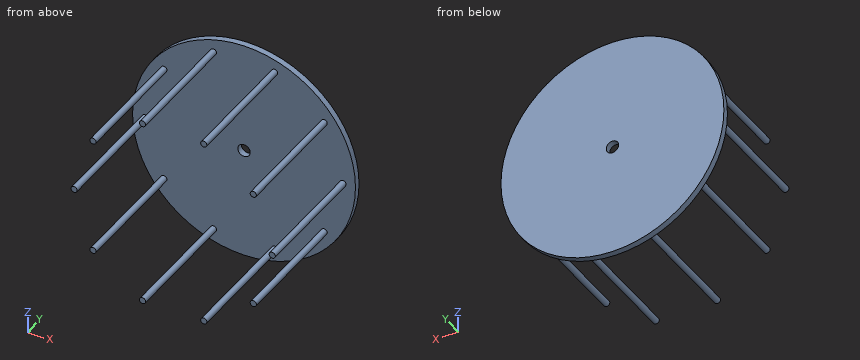
from build123d import *

# Parameters (mm, degrees)
F0_R     = 114.3
F0_R_2   = 6.35
F1_DEPTH = 6.35
F2_R     = 3.175
F3_DEPTH = 127


with BuildPart() as f1:
    # F0 (on Front) → F1 (new body)
    with BuildSketch(Plane.XZ):
        Circle(F0_R)
        Circle(F0_R_2, mode=Mode.SUBTRACT)
    extrude(amount=F1_DEPTH)

    # F2 (on face) → F3 (join)
    with BuildSketch(Plane.XZ.offset(6.35)):
        with Locations((101.6, 0)):
            Circle(F2_R)
        with Locations((82.196127, 59.718982)):
            Circle(F2_R)
        with Locations((31.396127, 96.627342)):
            Circle(F2_R)
        with Locations((-31.396127, 96.627342)):
            Circle(F2_R)
        with Locations((-82.196127, 59.718982)):
            Circle(F2_R)
        with Locations((-101.6, 0)):
            Circle(F2_R)
        with Locations((-82.196127, -59.718982)):
            Circle(F2_R)
        with Locations((-31.396127, -96.627342)):
            Circle(F2_R)
        with Locations((31.396127, -96.627342)):
            Circle(F2_R)
        with Locations((82.196127, -59.718982)):
            Circle(F2_R)
    extrude(amount=F3_DEPTH)


solid = f1.part
Verification items for the finished model (mm, model axes). Give positions to 0.01 mm unless a question says otherwise; leave off trailing zeros. Loops run counter-clockwise (first coordinate to the right, second up) from the corner with the lowest first, then second, coordinate; pieces in that order, holes last.
1) Depth check by flat-ended pin: pin 1 Ø4 at (x, z) = (-78, 17) entering from -Y. Enter the tip coordinate at first touch or a pass-through.
2) Sectioned sample at C-C, the plane y = -22. Count the separate pieces of the cut face and the enclosed holes in it, then the cut area to 3 significant figures.
3) Sectioned sample at B-B, the plane z = 0. Enter the section's corners in (x, y) (3 decimals).
4) Sectioned sample at A-A, the plane x = 0. Enter the section's corners in (y, z), then the cut area to 3 significant figures.
5) Thickness scan on line 1 along Z through (x, y) = (0, -4); line 2 along Y through (x, z) = (100.5, 7); line 3 along Z through (x, y) = (103.5, -14.5). Record the ranges inside material, lowest first.
6) Sectioned sample at D-D, the plane x = -101.6. Enter the section's corners in (y, z) (3 decimals).
Answers:
1. pin 1: stops at y = -6.35
2. separate pieces: 10
2. enclosed holes: 0
2. area: 317 mm2
3. outline: (-114.3, -6.35) - (-104.775, -6.35) - (-104.775, -133.35) - (-98.425, -133.35) - (-98.425, -6.35) - (-6.35, -6.35) - (-6.35, 0) - (-114.3, 0) - close; (6.35, -6.35) - (98.425, -6.35) - (98.425, -133.35) - (104.775, -133.35) - (104.775, -6.35) - (114.3, -6.35) - (114.3, 0) - (6.35, 0) - close
4. outline: (-6.35, -114.3) - (0, -114.3) - (0, -6.35) - (-6.35, -6.35) - close; (-6.35, 6.35) - (0, 6.35) - (0, 114.3) - (-6.35, 114.3) - close
4. area: 1,370 mm2
5. line 1: z = -114.3 to -6.35, 6.35 to 114.3
5. line 2: y = -6.35 to 0
5. line 3: z = -2.54 to 2.54
6. outline: (-133.35, -3.175) - (-6.35, -3.175) - (-6.35, -52.363) - (0, -52.363) - (0, 52.363) - (-6.35, 52.363) - (-6.35, 3.175) - (-133.35, 3.175) - close
